from build123d import *

# Parameters (mm, degrees)
F1_DEPTH = 10
F2_R     = 5


with BuildPart() as f1:
    # F0 (on Front) → F1 (new body, symmetric)
    with BuildSketch(Plane.XZ):
        with BuildLine():
            Line((-30.288021, 250.545293), (-111.82384, -27.369829))
            ThreePointArc((-111.82384, -27.369829), (-108.174209, -47.551816), (-89.827259, -56.718156))
            Line((-89.827259, -56.718156), (693.757768, -55.979899))
            ThreePointArc((693.757768, -55.979899), (783.507042, -18.730212), (820.672154, 71.054117))
            Line((820.672154, 71.054117), (820.672154, 454.555666))
            ThreePointArc((820.672154, 454.555666), (790.670941, 516.243982), (723.621847, 530.733294))
            Line((723.621847, 530.733294), (104.508811, 379.338224))
            ThreePointArc((104.508811, 379.338224), (19.883125, 332.972107), (-30.288021, 250.545293))
        make_face()
    extrude(amount=F1_DEPTH, both=True)

    # F2
    f2_edges = [f1.edges().sort_by_distance(p)[0] for p in [
        (19.883125, -10, 332.972107),
        (414.065329, -10, 455.035759),
        (790.670941, -10, 516.243982),
        (820.672154, -10, 262.804891),
        (783.507042, -10, -18.730212),
        (301.965255, -10, -56.349027),
        (-108.174209, 10, -47.551816),
        (-71.055931, -10, 111.587732),
        (-71.055931, 10, 111.587732),
        (19.883125, 10, 332.972107),
        (301.965255, 10, -56.349027),
    ]]
    fillet(f2_edges, radius=F2_R)


solid = f1.part
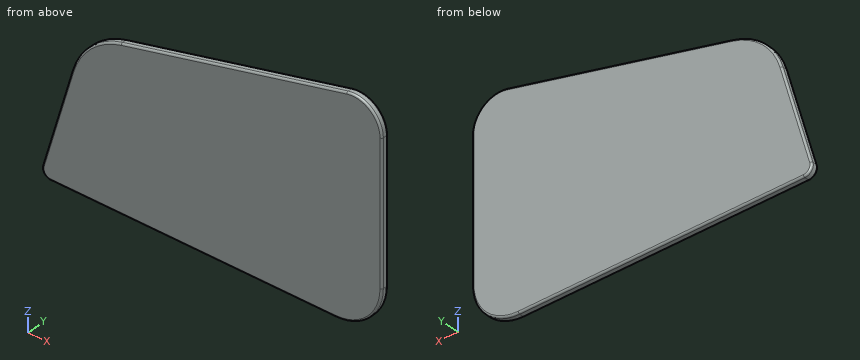
Model file for the job. Use its own axes, mm. Coordinates: 2 decimals unless noted, no trailing zeros. Order: outer loops, then holes, each group sorted by start corner. A loop starts at its lowest first (then second) coordinate and runs counter-clockwise, first axis right, second up. Notation, with made-up numbers: (30, 51) -> (37, 51) arc R27 ccw to (37, 87) -> close; hole circle Ø9 at (82, 33). An arc over 180 degrees is marked (long way). Return JSON: item names as keys, results as strings. Group by question number.
Item 1: Saw through at A-A on y = -1.75. Write the cut outline in (x, z).
Item 2: Wall check: line 1 along Y through (x, z) = (-63.5, 122.5); line 2 along Z through (x, y) = (730, 7.75); line 3 along X through (y, z) = (-3.5, 355.5). Give the ranges that are in metal, low to high. Write a range as [from, to].
Item 3: Flat gauge pins, fed straight in: P1, Ø8, axis at x = 52.5, y = 1, coming from the +Z side; P2, Ø1, axis at x = 465, y = -0.5, coming from the +Z side; P3, Ø2, axis at x = 300, y = -4.5, coming from the -Z side. Where does each tip first touch, or does it go through?
Values found:
{
 "1": {"outline": "(-111.82, -27.37) arc R22.9 ccw to (-89.83, -56.72) -> (693.76, -55.98) arc R127.03 ccw to (820.67, 71.05) -> (820.67, 454.56) arc R78.42 ccw to (723.62, 530.73) -> (104.51, 379.34) arc R186.69 ccw to (-30.29, 250.55) -> close"},
 "2": {"line 1": "y = [-9.93, 9.93]", "line 2": "z = [-49.8, 531.18]", "line 3": "x = [48.63, 820.67]"},
 "3": {"P1": "stops at z = 360.24", "P2": "stops at z = 467.61", "P3": "stops at z = -56.35"}
}
